Here's how the part is built. I have some questions about the finished solid (model axes, mm). Face numbers are marked on the shaded views. A direction names the side the tool comes from. Coordinates: 2 decimals unless noted, no trailing zeros. Order: outer loops, then holes, each group sorted by start corner. A loop starts at its lowest first (then second) coordinate and runs counter-clockwise, first axis right, second up.
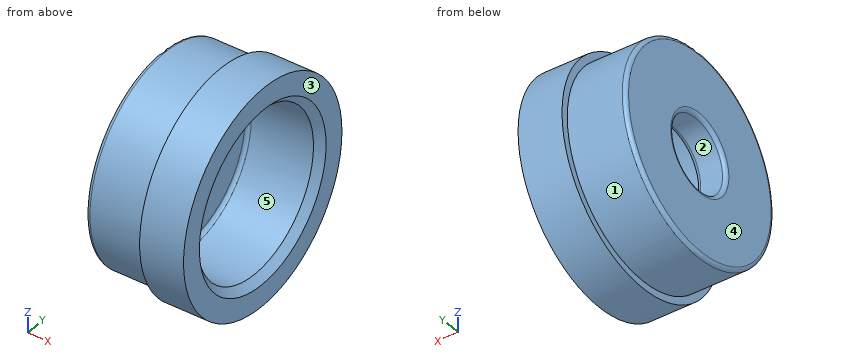
```python
from build123d import *

# Parameters (mm, degrees)
REDONDEO1_R   = 0.5
CHAFL_N1_SIZE = 1


with BuildPart() as part:
    # Croquis1 → Revolución1 (revolve)
    with BuildSketch(Plane.XY):
        Polygon((0, 11), (10, 11), (10, 14), (10, 15), (4, 15), (4, 14), (-4, 14), (-4, 5), (0, 5), align=None)
    revolve(axis=Axis((-5.995381062, 0, 0), (1, 0, 0)))

    # Redondeo1
    redondeo1_edges = [part.edges().sort_by_distance(p)[0] for p in [
        (0, -11, 0),
        (0, -5, 0),
        (-4, -5, 0),
        (-4, -14, 0),
    ]]
    fillet(redondeo1_edges, radius=REDONDEO1_R)

    # Chaflán1
    chafl_n1_edges = [part.edges().sort_by_distance(p)[0] for p in [
        (10, -11, 0),
    ]]
    chamfer(chafl_n1_edges, length=CHAFL_N1_SIZE)


solid = part.part
```
Q1. For the marked faces 4 and 5, which set-ups out of +Z, -Z, +X, -X, +Y, -Y let a thin tool reach every point of the face, with its end or its side?
Q2. We'd pull the mould along Z, two halves only. Please class the marked faces 1, 2 and 3: pulls with the +Z half, pulls with the -Z half, needs draft (parallel to the pull), parting line crosses it, or undercut.
Q3. If we section it at D-D on x = 7: Write out the boundary of the cut face in (y, z), then the cut area to 3 significant figures.
Q4. If we section it at A-A on z = 0: Write out the boundary of the cut face in (x, y), then the cut area to 3 significant figures.
Q5. Will these pins go through, and if not, where does the flat tip stop? pin 1 (6 mm diameter, centred on x = -1.5, y = -1, fed in from +Z); pin 2 (2 mm diameter, centred on x = 2, y = -9, fed in from -Z); pin 3 (17.5 mm diameter, centred on y = 0, z = 0, fed in from +X); pin 4 (6 mm diameter, centred on y = 0, z = 0, fed in from +X).
Q6. If we section it at C-C on x = 2: Write out the boundary of the cut face in (y, z), then the cut area to 3 significant figures.
Q7. I need wall thicknesses on L1, parallel to Z at x = -2.4, y = 0; L2, parallel to Z at x = 3.5, y = 0; L3, parallel to X at y = 2, z = 9.75. Which ranges of each line are inside material? Lowest first, please.
Reply:
1. face 4: +Z, -Z, -X, +Y, -Y
1. face 5: +X
2. face 1: parting line crosses it
2. face 2: undercut
2. face 3: needs draft
3. outline: circle Ø30 at (0, 0); hole circle Ø22 at (0, 0)
3. area: 327 mm2
4. outline: (-4, -13.5) arc R0.5 ccw to (-3.5, -14) - (4, -14) - (4, -15) - (10, -15) - (10, -12) - (9, -11) - (0.5, -11) arc R0.5 cw to (0, -10.5) - (0, -5.5) arc R0.5 ccw to (-0.5, -5) - (-3.5, -5) arc R0.5 ccw to (-4, -5.5) - close; (-4, 5.5) arc R0.5 ccw to (-3.5, 5) - (-0.5, 5) arc R0.5 ccw to (0, 5.5) - (0, 10.5) arc R0.5 cw to (0.5, 11) - (9, 11) - (10, 12) - (10, 15) - (4, 15) - (4, 14) - (-3.5, 14) arc R0.5 ccw to (-4, 13.5) - close
4. area: 143 mm2
5. pin 1: stops at z = 14
5. pin 2: stops at z = -11.49
5. pin 3: stops at x = 0
5. pin 4: passes through
6. outline: circle Ø28 at (0, 0); hole circle Ø22 at (0, 0)
6. area: 236 mm2
7. L1: z = -14 to -5, 5 to 14
7. L2: z = -14 to -11, 11 to 14
7. L3: x = -4 to 0
